Read the model definition and answer for the solid it produces. Units are mm, in the model's axes. A direction names the side the tool comes from. Round coordinates to 2 decimals unless told otherwise and drop trailing zeros. Loops run counter-clockwise (first coordinate to the right, second up) from the corner with the lowest first, then second, coordinate; pieces in that order, holes last. Notation, with made-up numbers: (30.5, 37) - (52.5, 37) arc R24 cw to (52.5, 63) - close; hole circle Ø1 at (6.25, 19). An arc over 180 degrees is marked (long way). Answer as CSV lines item,"result".
```python
from build123d import *

# Parameters (mm, degrees)
SKETCH1_W           = 27.3
SKETCH1_H           = 30
BOSS_EXTRUDE1_DEPTH = 6.35
SKETCH2_W           = 12.7
SKETCH2_H           = 6.35
BOSS_EXTRUDE2_DEPTH = 6.35
CUT_EXTRUDE1_DEPTH  = 7.35


with BuildPart() as part:
    # Sketch1 → Boss-Extrude1 (new body)
    with BuildSketch(Plane(origin=(0, 0, 0), x_dir=(1, 0, 0), z_dir=(0, 1, 0))):
        Rectangle(SKETCH1_W, SKETCH1_H)
    extrude(amount=BOSS_EXTRUDE1_DEPTH)

    # Sketch2 → Boss-Extrude2 (add)
    with BuildSketch(Plane(origin=(13.65, 0, 0), x_dir=(0, 0, -1), z_dir=(1, 0, 0))):
        with Locations((0, 3.175)):
            Rectangle(SKETCH2_W, SKETCH2_H)
    boss_extrude2 = extrude(amount=BOSS_EXTRUDE2_DEPTH)

    # Mirror1: Boss-Extrude2 across plane
    add(boss_extrude2.mirror(Plane(origin=(0, 0, 0), x_dir=(0, 0, 1), z_dir=(1, 0, 0))))

    # Sketch3 → Cut-Extrude1 (cut, through all)
    with BuildSketch(Plane(origin=(0, 6.35, 0), x_dir=(1, 0, 0), z_dir=(0, 1, 0))):
        with BuildLine():
            Line((-9.15, -7.917543811), (-9.15, 7.917543811))
            ThreePointArc((-9.15, 7.917543811), (0, 12.1), (9.15, 7.917543811))
            Line((9.15, 7.917543811), (9.15, -7.917543811))
            ThreePointArc((9.15, -7.917543811), (0, -12.1), (-9.15, -7.917543811))
        make_face()
    extrude(amount=-CUT_EXTRUDE1_DEPTH, mode=Mode.SUBTRACT)


solid = part.part
```
1) Each of these flat-tipped pins is pushed along its axis until it touches: P1, Ø10, axis at x = 1.5, z = -6.5, coming from the +Y side; P2, Ø3, axis at y = 2, z = -9, coming from the -X side; P3, Ø1.9, axis at y = 2.5, z = 11.5, coming from the +X side; P4, Ø1.9, axis at x = 16, y = 2, coming from the +Z side. Where does it stop, or does it pass through?
Entries:
P1,"passes through"
P2,"stops at x = -13.65"
P3,"stops at x = 13.65"
P4,"stops at z = 6.35"
2) A cutting plane is placed at C-C, the plane y = 1. Determine the outline of the cut face in (x, z).
Entries:
outline,"(-20, -6.35) - (-13.65, -6.35) - (-13.65, -15) - (13.65, -15) - (13.65, -6.35) - (20, -6.35) - (20, 6.35) - (13.65, 6.35) - (13.65, 15) - (-13.65, 15) - (-13.65, 6.35) - (-20, 6.35) - close; hole (-9.15, -7.92) arc R12.1 ccw to (9.15, -7.92) - (9.15, 7.92) arc R12.1 ccw to (-9.15, 7.92) - close"
3) A tool of negligible diameter and unlimited length cuts with its end or side. For faces 4 (the face through (-0.1, 3.2, -12.1)), 5 (the face through (-17, 3, 6.35)), 6 (the face through (-13.65, 3, -11)), 7 (the face through (17, 3, -6.35)), from which of +Z, -Z, +X, -X, +Y, -Y can it reach the whole face along a straight path? Write none if from no direction.
Entries:
face 4,"+Y, -Y"
face 5,"+Z, -X, +Y, -Y"
face 6,"-Z, -X, +Y, -Y"
face 7,"-Z, +X, +Y, -Y"
4) A cutting plane is placed at A-A, the plane z = 7. Determine the outline of the cut face in (x, y).
Entries:
outline,"(-13.65, 0) - (-9.15, 0) - (-9.15, 6.35) - (-13.65, 6.35) - close; (9.15, 0) - (13.65, 0) - (13.65, 6.35) - (9.15, 6.35) - close"
5) A cutting plane is placed at B-B, the plane x = 3. Determine the outline of the cut face in (y, z).
Entries:
outline,"(0, -15) - (6.35, -15) - (6.35, -11.72) - (0, -11.72) - close; (0, 11.72) - (6.35, 11.72) - (6.35, 15) - (0, 15) - close"
6) The mould has two halves that part along X. Classify faces 1 (the face through (0.1, 3.2, 12.1)), 2 (the face through (-13.65, 3, 11)), 3 (the face through (13.65, 3, 11)): pulls with the +X half, pulls with the -X half, needs draft (parallel to the pull), parting line crosses it, or undercut.
Entries:
face 1,"undercut"
face 2,"pulls with the -X half"
face 3,"pulls with the +X half"
7) Find the intervals of material crossed by line 1 (X direction, y = 6.25, z = -2); line 2 (X direction, y = 3, z = 7); line 3 (X direction, y = 0.75, z = 12.25), in increasing order.
Entries:
line 1,"x = -20 to -9.15, 9.15 to 20"
line 2,"x = -13.65 to -9.15, 9.15 to 13.65"
line 3,"x = -13.65 to 13.65"
8) A cutting plane is placed at D-D, the plane x = 15. Determine the outline of the cut face in (y, z), plus the area to 3 significant figures.
Entries:
outline,"(0, -6.35) - (6.35, -6.35) - (6.35, 6.35) - (0, 6.35) - close"
area,"80.6 mm^2"
